from build123d import *

# Parameters (mm, degrees)
STOCK_VARAV_UKSEGA_1_START = 312
STOCK_VARAV_UKSEGA_1_DEPTH = 10
TAB1_START                 = -10
SKETCH1_R                  = 7.5
TAB1_DEPTH                 = 10


# Read off the part's stored shape, not the designer's step: Stock-Varav_uksega-1
# Sheet-metal steps are written as plain solids
with BuildPart() as part:
    # Stock-Varav_uksega-1 outline → Stock-Varav_uksega-1 (new body)
    with BuildSketch(Plane(origin=(0, 0, 0), x_dir=(1, 0, 0), z_dir=(0, 1, 0)).offset(STOCK_VARAV_UKSEGA_1_START)):
        with BuildLine():
            Line((-11, 20), (-11, 50.267826876))
            ThreePointArc((-11, 50.267826876), (-12.117692031, 47.738612787), (-12.5, 45))
            Line((-12.5, 45), (-12.5, 20))
            Line((-12.5, 20), (-11, 20))
        make_face()
    extrude(amount=STOCK_VARAV_UKSEGA_1_DEPTH)

    # Sketch1 → Tab1 (add)
    with BuildSketch(Plane(origin=(0, 322, 0), x_dir=(1, 0, 0), z_dir=(0, 1, 0)).offset(TAB1_START)):
        with BuildLine():
            Line((-12.5, 20), (12.5, 20))
            Line((12.5, 20), (12.5, 45))
            ThreePointArc((12.5, 45), (9.571067812, 52.071067812), (2.5, 55))
            Line((2.5, 55), (-2.5, 55))
            ThreePointArc((-2.5, 55), (-9.571067812, 52.071067812), (-12.5, 45))
            Line((-12.5, 45), (-12.5, 20))
        make_face()
        with Locations(Location((0, 45, 0), (0, 0, 270))):
            Circle(SKETCH1_R, mode=Mode.SUBTRACT)
    extrude(amount=TAB1_DEPTH)


solid = part.part
Part model, mm, in its own coordinate system. Give positions to 0.01 mm unless a question says otherwise; leave off trailing zeros. Loops run counter-clockwise (first coordinate to the right, second up) from the corner with the lowest first, then second, coordinate; pieces in that order, holes last. Notation, with made-up numbers: (32.5, 28.5) -> (61.5, 28.5) arc R15 ccw to (61.5, 41.5) -> close; hole circle Ø5 at (-17, 74.25). An arc over 180 degrees is marked (long way). Write each question's results on one line, items separated by ' | '. Start each with the question number.
Q1. Band-saw the part on C-C on z = -44.5. List the corners of the cut face in (x, y), plus the area to 3 significant figures.
Q2. Pin check, flat tips, straight feed: P1, Ø13.5, axis at x = 0, z = -45, coming from the -Y side; P2, Ø8, axis at x = -3, z = -47.5, coming from the -Y side; P3, Ø1.5, axis at y = 318, z = -50.5, coming from the -X side; P4, Ø1.5, axis at x = -4, y = 317, coming from the -Z side. Stop position of each tip, or through.
Q3. Wall check: L1, parallel to X at y = 314, z = -45; L2, parallel to Z at x = -5.5, y = 318.25; L3, parallel to Z at x = -3.25, y = 313.25. Give the ranges that are in metal, low to high.
Q4. Pull direction Z, two halves, no side cores. Call faces 1 (the face through (0, 312, -34)), 2 (the face through (2.253, 316.93, -37.846)), 3 (the face through (9.65, 316.93, -51.99)): +Z half, -Z half, draft (parallel to the pull), parting line (faces both ways), or undercut.
Q5. Band-saw the part on A-A on y = 318.5. List the corners of the cut face in (x, z), plus the area to 3 significant figures.
Q6. Band-saw the part on D-D on x = -9.5. List the corners of the cut face in (y, z).
Q7. Band-saw the part on B-B on x = 0. List the corners of the cut face in (y, z), plus the area to 3 significant figures.
Results are:
1) outline: (-12.5, 312) -> (-7.48, 312) -> (-7.48, 322) -> (-12.5, 322) -> close; (7.48, 312) -> (12.5, 312) -> (12.5, 322) -> (7.48, 322) -> close | area: 100 mm²
2) P1: passes through | P2: stops at y = 312 | P3: stops at x = -11.3 | P4: stops at z = -54.97
3) L1: x = -12.5 to -7.5, 7.5 to 12.5 | L2: z = -54.54 to -50.1, -39.9 to -20 | L3: z = -54.97 to -51.76, -38.24 to -20
4) face 1: draft | face 2: undercut | face 3: -Z half
5) outline: (-12.5, -45) arc R10 ccw to (-2.5, -55) -> (2.5, -55) arc R10 ccw to (12.5, -45) -> (12.5, -20) -> (-12.5, -20) -> close; hole circle Ø15 at (0, -45) | area: 655 mm²
6) outline: (312, -52.14) -> (322, -52.14) -> (322, -20) -> (312, -20) -> close
7) outline: (312, -55) -> (322, -55) -> (322, -52.5) -> (312, -52.5) -> close; (312, -37.5) -> (322, -37.5) -> (322, -20) -> (312, -20) -> close | area: 200 mm²
